```python
from build123d import *

# Parameters (mm, degrees)
F0_W     = 2.9464
F0_H     = 3.556
F1_DEPTH = 13.9954
F0_H_2   = 26.3652
F2_DEPTH = 2.794
F3_DEPTH = 13.8684
F0_W_2   = 22.479
F0_H_3   = 2.9464
F4_DEPTH = 7.874


with BuildPart() as f1:
    # F0 (on Front) → F1 (new body)
    with BuildSketch(Plane.XZ):
        with Locations((-5.823712, 28.1432)):
            Rectangle(F0_W, F0_H)
        with Locations((31.184088, 28.1432)):
            Rectangle(F0_W, F0_H)
    extrude(amount=-F1_DEPTH)

    # F0 (on Front) → F2 (join)
    with BuildSketch(Plane.XZ):
        with Locations((-5.823712, 13.1826)):
            Rectangle(F0_W, F0_H_2)
        with Locations((31.184088, 13.1826)):
            Rectangle(F0_W, F0_H_2)
    extrude(amount=-F2_DEPTH)

    # F0 (on Front) → F3 (join)
    with BuildSketch(Plane.XZ):
        Polygon((32.657288, -15.7988), (32.657288, 0), (29.710888, 0), (23.919688, 0), (23.919688, -2.9464), (29.710888, -2.9464), (29.710888, -12.8524), (23.183088, -12.8524), (25.367488, -15.7988), (29.710888, -15.7988), align=None)
        Polygon((1.440688, -2.9464), (1.440688, 0), (-4.350512, 0), (-7.296912, 0), (-7.296912, -15.7988), (-4.350512, -15.7988), (0, -15.7988), (2.177288, -12.8524), (-4.350512, -12.8524), (-4.350512, -2.9464), align=None)
    extrude(amount=-F3_DEPTH)

    # F0 (on Front) → F4 (join)
    with BuildSketch(Plane.XZ):
        with Locations((12.680188, -1.4732)):
            Rectangle(F0_W_2, F0_H_3)
    extrude(amount=-F4_DEPTH)


solid = f1.part
```
Here's how the part is built. I have some questions about the finished solid (model axes, mm). A direction names the side the tool comes from. Round coordinates to 2 decimals unless told otherwise and drop trailing zeros. Loops run counter-clockwise (first coordinate to the right, second up) from the corner with the lowest first, then second, coordinate; pieces in that order, holes last. Notation, with made-up numbers: (32, 22.25) -> (41, 22.25) arc R35 ccw to (41, 55.25) -> close; hole circle Ø1 at (-18.75, 13.5). An arc over 180 degrees is marked (long way). Answer as CSV lines item,"result".
1. If I drill on L1, parallel to Z at x = 29, y = 6.5; L2, parallel to X at y = 1, z = 12.5; L3, parallel to Z at x = 31.5, y = 10.5, over which ranges is the centre line in solid material (lowest first)?
Final values:
L1,"z = -15.8 to -12.85, -2.95 to 0"
L2,"x = -7.3 to -4.35, 29.71 to 32.66"
L3,"z = -15.8 to 0, 26.37 to 29.92"
2. If we section it at B-B on y = 6.25: Please give me the cut outline in (x, z).
Final values:
outline,"(-7.3, -15.8) -> (0, -15.8) -> (2.18, -12.85) -> (-4.35, -12.85) -> (-4.35, -2.95) -> (29.71, -2.95) -> (29.71, -12.85) -> (23.18, -12.85) -> (25.37, -15.8) -> (32.66, -15.8) -> (32.66, 0) -> (-7.3, 0) -> close; (-7.3, 26.37) -> (-4.35, 26.37) -> (-4.35, 29.92) -> (-7.3, 29.92) -> close; (29.71, 26.37) -> (32.66, 26.37) -> (32.66, 29.92) -> (29.71, 29.92) -> close"
3. For pin 1 (4 mm diameter, centred on x = 19.5, y = 9.5, fed in from +Z); pin 2 (5 mm diameter, centred on x = 5.5, y = 10, fed in from -Z); pin 3 (1.5 mm diameter, centred on x = 20.5, y = 10.5, fed in from -Z); pin 4 (1.5 mm diameter, centred on x = 31, z = 9.5, fed in from +Y), each with a flat end and sliding along its axis, tell me the tip position at first contact or that it passes through.
Final values:
pin 1,"stops at z = 0"
pin 2,"stops at z = -2.95"
pin 3,"passes through"
pin 4,"stops at y = 2.79"
4. If we section it at D-D on y = 10.25: Please give me the cut outline in (x, z).
Final values:
outline,"(-7.3, -15.8) -> (0, -15.8) -> (2.18, -12.85) -> (-4.35, -12.85) -> (-4.35, -2.95) -> (1.44, -2.95) -> (1.44, 0) -> (-7.3, 0) -> close; (-7.3, 26.37) -> (-4.35, 26.37) -> (-4.35, 29.92) -> (-7.3, 29.92) -> close; (23.18, -12.85) -> (25.37, -15.8) -> (32.66, -15.8) -> (32.66, 0) -> (23.92, 0) -> (23.92, -2.95) -> (29.71, -2.95) -> (29.71, -12.85) -> close; (29.71, 26.37) -> (32.66, 26.37) -> (32.66, 29.92) -> (29.71, 29.92) -> close"
5. If we section it at C-C on x = 26: Please give me the cut outline in (y, z).
Final values:
outline,"(0, -15.8) -> (13.87, -15.8) -> (13.87, -12.85) -> (0, -12.85) -> close; (0, -2.95) -> (13.87, -2.95) -> (13.87, 0) -> (0, 0) -> close"
6. Which directions (+Z, -Z, +X, -X, +Y, -Y) give clear straight access to the entire face, cutting with the end or side of a thin tool? Please do faces 1 (the face through (-1, 7, -12.852)), 2 (the face through (24.26, 6.837, -14.305)), 3 (the face through (-5, 13.868, -8)).
Final values:
face 1,"+Y, -Y"
face 2,"-Z, +Y, -Y"
face 3,"-Z, +X, -X, +Y"
7. Thinking about a two-plate mould opening in X: for faces 4 (the face through (29.711, 2, 19)), 5 (the face through (23.92, 11, -1)), 6 (the face through (31, 8, 26.365)), which applies, released by +X, released by -X, zero draft, split by the parting line, or undercut?
Final values:
face 4,"undercut"
face 5,"undercut"
face 6,"zero draft"
8. If we section it at A-A on z = 27: Please give me the cut outline in (x, y), plus the area to 3 significant figures.
Final values:
outline,"(-7.3, 0) -> (-4.35, 0) -> (-4.35, 14) -> (-7.3, 14) -> close; (29.71, 0) -> (32.66, 0) -> (32.66, 14) -> (29.71, 14) -> close"
area,"82.5 mm^2"
